Solid Edge part; units mm, degrees
sketch "Sketch1" plane through (0, 0, 0) normal (0, -1, 0) x (1, 0, 0)
  line L0 (45, -40) -> (0, -40)
  line L1 (0, 40) -> (0, -40)
  line L2 (0, 40) -> (45, 40)
  line L3 (45, 40) -> (45, 37.4928)
  arc A0 (41.3486, 33.508) -> (45, 37.4928) centre (41, 37.4928) ccw
  line L4 (41.3486, 33.508) -> (13.3028, 31.0543)
  arc A1 (13.3028, 31.0543) -> (6, 23.0847) centre (14, 23.0847) ccw
  line L5 (6, -23.0847) -> (6, 23.0847)
  arc A2 (6, -23.0847) -> (13.3028, -31.0543) centre (14, -23.0847) ccw
  line L6 (41.3486, -33.508) -> (13.3028, -31.0543)
  arc A3 (41.3486, -33.508) -> (45, -37.4928) centre (41, -37.4928) cw
  line L7 (45, -40) -> (45, -37.4928)
extrude "Protrusion1" add sketch "Sketch1" against normal blind 28.575
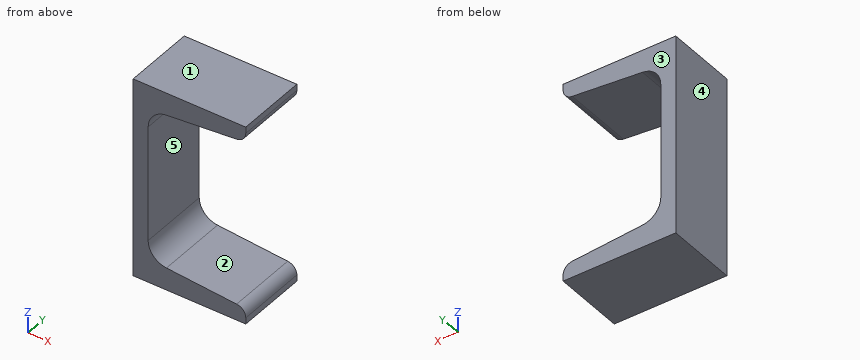
Geometry: final body of the model. Coordinates: model frame, mm. Face numbers are marked on the shaded views. A direction names the side the tool comes from. Coordinates: 2 decimals unless noted, no trailing zeros. Write each loop counter-clockwise with the first axis right and the second up, starting at its lowest first coordinate (ties: lowest second). Pieces come first, ordered by that corner, then holes. Notation, with made-up numbers: M -19.5,-19.5 L 3.5,-19.5 A28 cw 3.5,7.5 Z; hole C 34,21.5 d5. An arc over 180 degrees is marked long. Use CSV: the item, a comma, the result in double quotes. Start each with the question number.
1. Mould query, pull axis Z, two halves, no side actions, for the marked faces 1, 2 and 3. Classes: pulls with the +Z half, pulls with the -Z half, needs draft (parallel to the pull), parting line crosses it, or undercut.
2. Cut plane C-C on x = 36.5. Return the cut outline in (y, z) (3 decimals), plus the area to 3 significant figures.
3. Ray query, probe 1 along X at (y, z) = (20, -20.5); probe 2 along Z at (x, y) = (8.5, 16.5); probe 3 along Z at (x, y) = (22.5, 21). Return the intervals inside material, ascending.
4. Cut plane B-B on y = 18.5. Return the cut outline in (x, z), plus the area to 3 significant figures.
5. Reachability of the marked faces 4 and 5 from +Z, -Z, +X, -X, +Y, -Y: full face, straight path, thin tool, end or side. Return the list, or none.
6. Cut plane A-A on x = 30.5. Return the cut outline in (y, z) (3 decimals), plus the area to 3 significant figures.
7. Cut plane D-D on z = 21.5. Return the cut outline in (x, y) (3 decimals).
8. First-contact query: P1, Ø14.5, axis at y = 11, z = 5, coming from the +X side; P2, Ø1, axis at y = 3.5, z = -32, coming from the -X side. Flat tips, straight axial feed; report the tip coordinate or a pass-through.
Entries:
1,face 1,"pulls with the +Z half"
1,face 2,"undercut"
1,face 3,"needs draft"
2,outline,"M 0,-40 L 28.575,-40 L 28.575,-33.084 L 0,-33.084 Z; M 0,33.084 L 28.575,33.084 L 28.575,40 L 0,40 Z"
2,area,"395 mm²"
3,probe 1,"0 to 6"
3,probe 2,"-40 to -28.89, 28.89 to 40"
3,probe 3,"-40 to -31.86, 31.86 to 40"
4,outline,"M 0,-40 L 45,-40 L 45,-37.49 A4 ccw 41.35,-33.51 L 13.3,-31.05 A8 cw 6,-23.08 L 6,23.08 A8 cw 13.3,31.05 L 41.35,33.51 A4 ccw 45,37.49 L 45,40 L 0,40 Z"
4,area,"1,110 mm²"
5,face 4,"+Z, -Z, -X, +Y, -Y"
5,face 5,"+X, +Y, -Y"
6,outline,"M 0,-40 L 28.575,-40 L 28.575,-32.559 L 0,-32.559 Z; M 0,32.559 L 28.575,32.559 L 28.575,40 L 0,40 Z"
6,area,"425 mm²"
7,outline,"M 0,0 L 6,0 L 6,28.575 L 0,28.575 Z"
8,P1,"x = 6"
8,P2,"x = 0"
